Autodesk Inventor part; units mm, degrees
ref_plane "Work Plane1" through (-23.8699, -80.2202, 0) normal (0, 1, 0) x (-1, 0, 0)
ref_plane "YZ Plane" through (0, 0, 0) normal (1, 0, 0) x (0, 1, 0)
ref_plane "XY Plane" through (0, 0, 0) normal (0, 0, 1) x (1, 0, 0)
sketch "Sketch1" plane through (0, 0, 0) normal (0, 0, 1) x (1, 0, 0)
  arc A0 (-35.0421, -107.5967) -> (-23.9714, -112.0085) centre (-29.2466, -109.1496) ccw
  arc A1 (-27.3511, -78.8934) -> (27.3511, -78.8934) centre (0, 0) ccw
  line L0 (0, 0) -> (0, -147.6951) construction
  line L1 (0, 0) -> (-29.2466, -109.1496) construction
  line L2 (-35.0421, -107.5967) -> (-27.3511, -78.8934)
  arc A2 (0, -97.7345) -> (-23.9714, -112.0085) centre (0, -125) ccw
  arc A3 (23.9714, -112.0085) -> (35.0421, -107.5967) centre (29.2466, -109.1496) ccw
  line L3 (35.0421, -107.5967) -> (27.3511, -78.8934)
  arc A4 (23.9714, -112.0085) -> (0, -97.7345) centre (0, -125) ccw
  dimension "d0" = 167
  dimension "d1" = 12
  dimension "d2" = 15
  dimension "d3" = 113
  dimension "d4" = 125
extrude "Extrusion1" add sketch "Sketch1" along normal blind 6
sketch "Sketch2" plane through (0, 0, 6) normal (0, 0, 1) x (1, 0, 0)
  line L0 (-29.2466, -109.1496) -> (0, 0) construction
  line L1 (0, 0) -> (29.2466, -109.1496) construction
  line L2 (0, 0) -> (0, -137.2486) construction
  dimension "d14" = 15
  dimension "d15" = 15
  dimension "d16" = 113
  dimension "d17" = 113
hole "Hole1" at (-29.2466, -109.1496, 6) at (29.2466, -109.1496, 6) direction (0, 0, -1) diameter 4.5 end through all countersink diameter 9.4 countersink angle 90
fillet "Fillet1" radius 5 2 edges at (-27.3511, -78.8934, 3) (27.3511, -78.8934, 3)
ref_plane "Work Plane1" through (-23.8699, -80.2202, 0) normal (0, 1, 0) x (-1, 0, 0)
sketch "Sketch3" plane through (-23.8699, -80.2202, 0) normal (0, 1, 0) x (-1, 0, 0)
  line L0 (11.1722, 0) -> (11.1722, 6)
  point P0 (-23.8699, 0)
  point P1 (-23.8699, 3)
  point P2 (11.1722, 3)
hole "Hole2" at (0, -80.2202, 3) direction (0, -1, 0) diameter 4 end through all
sketch "Sketch4" plane through (0, 0, 6) normal (0, 0, 1) x (1, 0, 0)
  arc A0 (-22.5214, -80.4055) -> (22.5214, -80.4055) centre (0, 0) ccw
  circle A1 centre (0, -83.5) radius 3
  point P0 (0, -83.5)
  point P1 (0, -83.5)
  dimension "d26" = 6
extrude "Extrusion2" cut sketch "Sketch4" against normal through all
fillet "Fillet2" radius 5 2 edges at (-2.9995, -83.4461, 3) (2.9995, -83.4461, 3)
equation "\"d15\" = d14"
equation "\"d17\" = d16"
properties part number "Gradient_positioner"
The model under review builds one solid part; all positions refer to its coordinate system, in mm. A direction names the side the tool comes from. Round coordinates to 2 decimals unless told otherwise and drop trailing zeros. Loops run counter-clockwise (first coordinate to the right, second up) from the corner with the lowest first, then second, coordinate; pieces in that order, holes last.
Item 1: For faces 4 (the face through (31.915, -95.927, 2.958)), 5 (the face through (-14.13, -101.68, 2.96)), 6 (the face through (14.479, -82.235, 2.958)), list the 3-axis set-ups (+Z, -Z, +X, -X, +Y, -Y) from which the entire face can be reached by the end or side of a thin tool; tool diameter is ignored.
Determined:
face 4: +Z, -Z, +X, +Y
face 5: +Z, -Z, -Y
face 6: +Z, -Z, +Y
Item 2: Take a section at D-D (x = 19.5). Write out the cut boundary in (y, z), then the cut area to 3 significant figures.
Determined:
outline: (-105.94, 0) - (-81.19, 0) - (-81.19, 6) - (-105.94, 6) - close
area: 149 mm2
Item 3: Clearance check with flat-ended pins moving along their axes: pin 1 Ø2 at (x, z) = (-27, 4) entering from -Y; pin 2 Ø3.5 at (x, y) = (-29.25, -109.15) entering from +Z; pin 3 Ø6 at (x, y) = (29.25, -109.15) entering from +Z. State where each tip first meets the part, or that it passes through.
Determined:
pin 1: stops at y = -115.02
pin 2: passes through
pin 3: stops at z = 4.3
Item 4: For line 1 (X direction, y = -110, z = 0.5); line 2 (X direction, y = -85.5, z = 4.75); line 3 (X direction, y = -94.5, z = 3), list the stretches that pass through material, from the lowest coordinate up.
Determined:
line 1: x = -35.19 to -31.33, -27.16 to -22.77, 22.77 to 27.16, 31.33 to 35.19
line 2: x = -29.12 to -2.24, 2.24 to 29.12
line 3: x = -31.53 to -2, 2 to 31.53
Item 5: Take a section at C-C (x = 8). Write out the cut boundary in (y, z), then the cut area to 3 significant figures.
Determined:
outline: (-98.93, 0) - (-83.12, 0) - (-83.12, 6) - (-98.93, 6) - close
area: 94.9 mm2
Item 6: Take a section at A-A (z = 2.25). Give the number of separate pieces and of enclosed holes in the cut face, then the cut area to 3 significant figures.
Determined:
separate pieces: 2
enclosed holes: 2
area: 1,390 mm2
Item 7: Mouldability with a two-part tool opening along Y and no side actions: class faces 1 (the face through (-30.709, -107.242, 3.703)), 2 (the face through (0.766, -91.856, 4.847)), 3 (the face through (26.39, -80.9, 3.04)) as released by +Y, released by -Y, zero draft, split by the parting line, or undercut.
Determined:
face 1: undercut
face 2: zero draft
face 3: released by +Y
